```python
from build123d import *

# Parameters (mm, degrees)
SKETCH1_W                                            = 35.56
SKETCH1_H                                            = 20.574
BOSS_EXTRUDE1_DEPTH                                  = 12.7
SKETCH2_W                                            = 26.416
SKETCH2_H                                            = 11.43
CUT_EXTRUDE1_DEPTH                                   = 6.35
CBORE_FOR_5_16_TRUSS_HEAD_SCREW1_D                   = 3.175
CBORE_FOR_5_16_TRUSS_HEAD_SCREW1_DEPTH               = 7.9375
CBORE_FOR_5_16_TRUSS_HEAD_SCREW1_CBORE_D             = 6.35
CBORE_FOR_5_16_TRUSS_HEAD_SCREW1_CBORE_DEPTH         = 2.38125
CBORE_FOR_5_16_TRUSS_HEAD_SCREW1_TIP                 = 0.953866233
CBORE_FOR_5_16_TRUSS_HEAD_SCREW1_ON_FACE_D           = 3.175
CBORE_FOR_5_16_TRUSS_HEAD_SCREW1_ON_FACE_DEPTH       = 7.9375
CBORE_FOR_5_16_TRUSS_HEAD_SCREW1_ON_FACE_CBORE_D     = 6.35
CBORE_FOR_5_16_TRUSS_HEAD_SCREW1_ON_FACE_CBORE_DEPTH = 2.38125
CBORE_FOR_5_16_TRUSS_HEAD_SCREW1_ON_FACE_TIP         = 0.953866233
SKETCH5_W                                            = 4.572
SKETCH5_H                                            = 20.574
BOSS_EXTRUDE2_DEPTH                                  = 26.9748
CUT_EXTRUDE2_REACH                                   = 59.113
SKETCH7_W                                            = 11.9888
SKETCH7_H                                            = 22.8092
F_60_0_04_DIAMETER_HOLE1_D                           = 2.794
F_60_0_04_DIAMETER_HOLE1_DEPTH                       = 5.08
F_60_0_04_DIAMETER_HOLE1_TIP                         = 0.839402285
CUT_EXTRUDE3_REACH                                   = 59.113
SKETCH10_R                                           = 6.35
FILLET1_R                                            = 1.27


with BuildPart() as part:
    # Sketch1 → Boss-Extrude1 (new body)
    with BuildSketch(Plane(origin=(0, 0, 0), x_dir=(1, 0, 0), z_dir=(0, 1, 0))):
        with Locations((0, 10.287)):
            Rectangle(SKETCH1_W, SKETCH1_H)
    extrude(amount=BOSS_EXTRUDE1_DEPTH)

    # Sketch2 → Cut-Extrude1 (cut)
    with BuildSketch(Plane.XZ):
        with Locations((0, -10.287)):
            Rectangle(SKETCH2_W, SKETCH2_H)
    extrude(amount=-CUT_EXTRUDE1_DEPTH, mode=Mode.SUBTRACT)

    # CBORE for 5/16 Truss Head Screw1
    with Locations(Plane(origin=(-3.81, 12.7, -14.097), x_dir=(0, 0, 1), z_dir=(0, 1, 0))):
        with Locations((0, 0), (0, 7.62), (7.62, 0), (7.62, 7.62)):
            CounterBoreHole(CBORE_FOR_5_16_TRUSS_HEAD_SCREW1_D / 2, CBORE_FOR_5_16_TRUSS_HEAD_SCREW1_CBORE_D / 2, CBORE_FOR_5_16_TRUSS_HEAD_SCREW1_CBORE_DEPTH, depth=CBORE_FOR_5_16_TRUSS_HEAD_SCREW1_DEPTH)
            with Locations((0, 0, -(CBORE_FOR_5_16_TRUSS_HEAD_SCREW1_DEPTH + CBORE_FOR_5_16_TRUSS_HEAD_SCREW1_TIP / 2))):  # 118° drill point
                Cone(0, CBORE_FOR_5_16_TRUSS_HEAD_SCREW1_D / 2, CBORE_FOR_5_16_TRUSS_HEAD_SCREW1_TIP, mode=Mode.SUBTRACT)

    # CBORE for 5/16 Truss Head Screw1 on face
    with Locations(Plane(origin=(-4.806161328, 124.310596627, 0), x_dir=(0, 0, 1), z_dir=(0, 1, 0))):
        with Locations((0, 0)):
            CounterBoreHole(CBORE_FOR_5_16_TRUSS_HEAD_SCREW1_ON_FACE_D / 2, CBORE_FOR_5_16_TRUSS_HEAD_SCREW1_ON_FACE_CBORE_D / 2, CBORE_FOR_5_16_TRUSS_HEAD_SCREW1_ON_FACE_CBORE_DEPTH, depth=CBORE_FOR_5_16_TRUSS_HEAD_SCREW1_ON_FACE_DEPTH)
            with Locations((0, 0, -(CBORE_FOR_5_16_TRUSS_HEAD_SCREW1_ON_FACE_DEPTH + CBORE_FOR_5_16_TRUSS_HEAD_SCREW1_ON_FACE_TIP / 2))):  # 118° drill point
                Cone(0, CBORE_FOR_5_16_TRUSS_HEAD_SCREW1_ON_FACE_D / 2, CBORE_FOR_5_16_TRUSS_HEAD_SCREW1_ON_FACE_TIP, mode=Mode.SUBTRACT)

    # Sketch5 → Boss-Extrude2 (add)
    with BuildSketch(Plane(origin=(0, 12.7, 0), x_dir=(1, 0, 0), z_dir=(0, 1, 0))):
        with Locations((-15.494, 10.287)):
            Rectangle(SKETCH5_W, SKETCH5_H)
        with Locations((15.494, 10.287)):
            Rectangle(SKETCH5_W, SKETCH5_H)
    extrude(amount=BOSS_EXTRUDE2_DEPTH)

    # Sketch7 → Cut-Extrude2 (cut, up to next)
    with BuildSketch(Plane(origin=(17.78, 0, 0), x_dir=(0, 0, -1), z_dir=(1, 0, 0)), mode=Mode.PRIVATE) as cut_extrude2_sk1:
        with Locations((10.287, 24.1046)):
            Rectangle(SKETCH7_W, SKETCH7_H)
    cut_extrude2_tool1 = extrude(cut_extrude2_sk1.sketch, amount=-CUT_EXTRUDE2_REACH, mode=Mode.PRIVATE) & part.part
    add(cut_extrude2_tool1.solids().sort_by_distance((17.78, 24.1046, -10.287))[0], mode=Mode.SUBTRACT)

    # #60 (0.04) Diameter Hole1
    with Locations(Plane(origin=(17.78, 0, 0), x_dir=(0, 0, -1), z_dir=(1, 0, 0))):
        with Locations((10.287, 38.4048), (10.286762393, 9.906)):
            Hole(F_60_0_04_DIAMETER_HOLE1_D / 2, depth=F_60_0_04_DIAMETER_HOLE1_DEPTH)
            with Locations((0, 0, -(F_60_0_04_DIAMETER_HOLE1_DEPTH + F_60_0_04_DIAMETER_HOLE1_TIP / 2))):  # 118° drill point
                Cone(0, F_60_0_04_DIAMETER_HOLE1_D / 2, F_60_0_04_DIAMETER_HOLE1_TIP, mode=Mode.SUBTRACT)

    # Sketch10 → Cut-Extrude3 (cut, up to next)
    with BuildSketch(Plane.ZY.offset(17.78), mode=Mode.PRIVATE) as cut_extrude3_sk1:
        with Locations((-10.287, 29.464)):
            Circle(SKETCH10_R)
    cut_extrude3_tool1 = extrude(cut_extrude3_sk1.sketch, amount=-CUT_EXTRUDE3_REACH, mode=Mode.PRIVATE) & part.part
    add(cut_extrude3_tool1.solids().sort_by_distance((-17.78, 29.464, -10.287))[0], mode=Mode.SUBTRACT)

    # Fillet1
    fillet1_edges = [part.edges().sort_by_distance(p)[0] for p in [
        (17.78, 39.6748, -15.721493557),
        (13.208, 39.6748, -4.852506443),
        (-13.208, 0, -10.287),
        (0, 0, -16.002),
        (13.208, 0, -10.287),
        (0, 0, -4.572),
        (0, 0, -20.574),
        (17.78, 0, -10.287),
        (0, 0, 0),
        (-17.78, 0, -10.287),
        (0, 12.7, 0),
        (-13.208, 12.7, -10.287),
        (-13.208, 26.1874, 0),
        (-13.208, 26.1874, -20.574),
        (-17.78, 39.6748, -10.287),
        (-15.494, 39.6748, 0),
        (-13.208, 39.6748, -10.287),
        (-15.494, 39.6748, -20.574),
        (0, 12.7, -20.574),
        (-17.78, 19.8374, -20.574),
        (17.78, 19.8374, -20.574),
        (13.208, 26.1874, -20.574),
        (17.78, 19.8374, 0),
        (13.208, 26.1874, 0),
        (17.78, 39.6748, -4.852506443),
        (15.494, 39.6748, -20.574),
        (13.208, 39.6748, -15.721493557),
        (-17.78, 19.8374, 0),
        (15.494, 39.6748, 0),
        (13.208, 35.5092, -10.287),
        (13.208, 24.1046, -16.2814),
        (13.208, 24.1046, -4.2926),
        (17.78, 24.1046, -16.2814),
        (17.78, 35.5092, -10.287),
        (17.78, 24.1046, -4.2926),
    ]]
    fillet(fillet1_edges, radius=FILLET1_R)


solid = part.part
```
The listing builds one solid part. Answer for the finished solid, in the listing's coordinates (mm). A direction names the side the tool comes from. Coordinates: 2 decimals unless noted, no trailing zeros. Loops run counter-clockwise (first coordinate to the right, second up) from the corner with the lowest first, then second, coordinate; pieces in that order, holes last. Notation, with made-up numbers: (36, -0.75) -> (40, -0.75) arc R12 ccw to (40, 7.25) -> close; hole circle Ø6 at (1.5, -29.75). An arc over 180 degrees is marked (long way). Return JSON: item names as keys, results as strings. Group by question number.
(1) A cutting plane is placed at B-B on x = -3.81. Count the separate pieces of the cut face and the enclosed holes in it, and give its area (3 significant figures).
(2) A cutting plane is placed at D-D on y = 26.5. Write down the section's boundary in (x, z), and give its area (3 significant figures).
(3) A cutting plane is placed at A-A on y = 5.5. Write down the section's boundary in (x, z), and give its area (3 significant figures).
(4) Given pin 1 Ø5.5 at (x, z) = (3.81, -14.097) entering from -Y; pin 2 Ø3 at (x, z) = (2.5, -7) entering from +Y; pin 3 Ø5 at (x, y) = (11.5, 34.5) entering from +Z, each flat-ended and moving along its own axis, determine where each tip first touches the part or whether it passes through.
(5) Find the intervals of material crossed by probe 1 along X at (y, z) = (9, -14.25); probe 2 along Z at (x, y) = (11.5, 3.5); probe 3 along X at (y, z) = (23, -2), in increasing order. Write a range as from..to.
(6) Determine the mould class of faces 1 (the cylindrical face through (17.42, 39.29, -15.15)), 2 (the cylindrical face through (-15.48, 39.313, -20.192)), 3 (the cylindrical face through (-13.59, 39.31, -10.41)) for opening direction X: released by +X, released by -X, zero draft, split by the parting line, or undercut.
(7) A cutting plane is placed at C-C on y = 22.5. Write down the section's boundary in (x, z), and give its area (3 significant figures).
(8) Which of the six approach directions +Z, -Z, +X, -X, +Y, -Y give full straight-line access (tool end or side, diameter ignored) to faces 4 (the flat face through (13.208, 28, -18)), 5 (the flat face through (5, 10.319, -8)), 6 (the flat face through (0, 4, -4.572)), 7 (the cylindrical face through (15.46, 37.01, -10.34))?
The answers:
{
 "1": {"separate pieces": "3", "enclosed holes": "0", "area": "131 mm^2"},
 "2": {"outline": "(-17.78, -19.3) arc R1.27 ccw to (-16.51, -20.57) -> (-14.48, -20.57) arc R1.27 ccw to (-13.21, -19.3) -> (-13.21, -15.9) -> (-17.78, -15.9) -> close; (-17.78, -4.67) -> (-13.21, -4.67) -> (-13.21, -1.27) arc R1.27 ccw to (-14.48, 0) -> (-16.51, 0) arc R1.27 ccw to (-17.78, -1.27) -> close; (13.21, -19.3) arc R1.27 ccw to (14.48, -20.57) -> (16.51, -20.57) arc R1.27 ccw to (17.78, -19.3) -> (17.78, -17.55) arc R1.27 ccw to (16.51, -16.28) -> (14.48, -16.28) arc R1.27 ccw to (13.21, -17.55) -> close; (13.21, -3.02) arc R1.27 ccw to (14.48, -4.29) -> (16.51, -4.29) arc R1.27 ccw to (17.78, -3.02) -> (17.78, -1.27) arc R1.27 ccw to (16.51, 0) -> (14.48, 0) arc R1.27 ccw to (13.21, -1.27) -> close", "area": "77.8 mm^2"},
 "3": {"outline": "(-17.78, -19.3) arc R1.27 ccw to (-16.51, -20.57) -> (16.51, -20.57) arc R1.27 ccw to (17.78, -19.3) -> (17.78, -1.27) arc R1.27 ccw to (16.51, 0) -> (-16.51, 0) arc R1.27 ccw to (-17.78, -1.27) -> close; hole (-13.21, -16) -> (13.21, -16) -> (13.21, -4.57) -> (-13.21, -4.57) -> close", "area": "428 mm^2"},
 "4": {"pin 1": "stops at y = 0.07", "pin 2": "stops at y = 10.32", "pin 3": "stops at z = -0.09"},
 "5": {"probe 1": "x = -17.78..-5.39, -2.23..2.23, 5.39..17.78", "probe 2": "z = -20.57..-16, -4.57..0", "probe 3": "x = -17.78..-13.21, 13.21..17.78"},
 "6": {"face 1": "released by +X", "face 2": "zero draft", "face 3": "undercut"},
 "7": {"outline": "(-17.78, -19.3) arc R1.27 ccw to (-16.51, -20.57) -> (-14.48, -20.57) arc R1.27 ccw to (-13.21, -19.3) -> (-13.21, -1.27) arc R1.27 ccw to (-14.48, 0) -> (-16.51, 0) arc R1.27 ccw to (-17.78, -1.27) -> close; (13.21, -19.3) arc R1.27 ccw to (14.48, -20.57) -> (16.51, -20.57) arc R1.27 ccw to (17.78, -19.3) -> (17.78, -17.55) arc R1.27 ccw to (16.51, -16.28) -> (14.48, -16.28) arc R1.27 ccw to (13.21, -17.55) -> close; (13.21, -3.02) arc R1.27 ccw to (14.48, -4.29) -> (16.51, -4.29) arc R1.27 ccw to (17.78, -3.02) -> (17.78, -1.27) arc R1.27 ccw to (16.51, 0) -> (14.48, 0) arc R1.27 ccw to (13.21, -1.27) -> close", "area": "129 mm^2"},
 "8": {"face 4": "+Z, -Z, +Y", "face 5": "+Y", "face 6": "-Y", "face 7": "+X"}
}
